Verification items for the finished model (mm, model axes). A direction names the side the tool comes from. Round coordinates to 2 decimals unless told otherwise and drop trailing zeros. Loops run counter-clockwise (first coordinate to the right, second up) from the corner with the lowest first, then second, coordinate; pieces in that order, holes last. Notation, with made-up numbers: M -32.5,31.25 L -25.5,31.25 A20 cw -25.5,64.25 Z; hole C 44,-14.5 d11. An arc over 180 degrees is marked long. One line per item, written item: value.
from build123d import *
from build123d.topology import SkipClean

# Parameters (mm, degrees)
SKETCH1_R           = 65
SKETCH1_R_2         = 5
SKETCH1_R_3         = 3
SKETCH1_R_4         = 1.55
BOSS_EXTRUDE1_DEPTH = 5
SKETCH2_R           = 14
CUT_EXTRUDE2_DEPTH  = 10
SKETCH3_R           = 2.25
SKETCH3_W           = 17.301764966
SKETCH3_H           = 25.534036418
CUT_EXTRUDE3_DEPTH  = 10
BOSS_EXTRUDE2_START = -27.5
SKETCH4_R           = 3
BOSS_EXTRUDE2_DEPTH = 22.5
SKETCH6_W           = 6
SKETCH6_H           = 20
CUT_EXTRUDE4_DEPTH  = 22.5
CUT_EXTRUDE5_REACH  = 101.575


with BuildPart() as part:
    # Sketch1 → Boss-Extrude1 (new body)
    with BuildSketch(Plane(origin=(0, 0, 0), x_dir=(1, 0, 0), z_dir=(0, 1, 0))):
        with Locations(Location((0, 0, 0), (0, 0, 270))):
            Circle(SKETCH1_R)
        with Locations(Location((0, 0, 0), (0, 0, 270))):
            Circle(SKETCH1_R_2, mode=Mode.SUBTRACT)
        with Locations(Location((0, 42.5, 0), (0, 0, 270))):
            Circle(SKETCH1_R_3, mode=Mode.SUBTRACT)
        with Locations(Location((42.5, 0, 0), (0, 0, 270))):
            Circle(SKETCH1_R_3, mode=Mode.SUBTRACT)
        with Locations(Location((0, -42.5, 0), (0, 0, 270))):
            Circle(SKETCH1_R_3, mode=Mode.SUBTRACT)
        with Locations(Location((-42.5, 0, 0), (0, 0, 270))):
            Circle(SKETCH1_R_3, mode=Mode.SUBTRACT)
        with Locations(Location((-42.5, -12.5, 0), (0, 0, 270))):
            Circle(SKETCH1_R_4, mode=Mode.SUBTRACT)
        with Locations(Location((-42.5, 12.5, 0), (0, 0, 270))):
            Circle(SKETCH1_R_4, mode=Mode.SUBTRACT)
        with Locations(Location((42.5, -12.5, 0), (0, 0, 90))):
            Circle(SKETCH1_R_4, mode=Mode.SUBTRACT)
        with Locations(Location((42.5, 12.5, 0), (0, 0, 90))):
            Circle(SKETCH1_R_4, mode=Mode.SUBTRACT)
    extrude(amount=BOSS_EXTRUDE1_DEPTH)

    # Sketch2 → Cut-Extrude2 (cut)
    with BuildSketch(Plane(origin=(0, 0, 0), x_dir=(-1, 0, 0), z_dir=(0, -1, 0))):
        with Locations(Location((-7.999467705, -0.092284522, 0), (0, 0, 90))):
            Circle(SKETCH2_R)
    extrude(amount=-CUT_EXTRUDE2_DEPTH, mode=Mode.SUBTRACT)

    # Sketch3 → Cut-Extrude3 (cut)
    with BuildSketch(Plane(origin=(0, 0, 0), x_dir=(-1, 0, 0), z_dir=(0, -1, 0))):
        with Locations(Location((-7.999467705, -17.592284522, 0), (0, 0, 90))):
            Circle(SKETCH3_R)
        with Locations(Location((-7.999467705, 17.407715478, 0), (0, 0, 90))):
            Circle(SKETCH3_R)
        with Locations((-18.812677283, 0)):
            Rectangle(SKETCH3_W, SKETCH3_H)
    extrude(amount=-CUT_EXTRUDE3_DEPTH, mode=Mode.SUBTRACT)

    # Sketch4 → Boss-Extrude2 (add)
    with BuildSketch(Plane(origin=(0, 5, 0), x_dir=(1, 0, 0), z_dir=(0, 1, 0)).offset(BOSS_EXTRUDE2_START)):
        Polygon((-7, 42.5), (-7, 22.5), (7, 22.5), (7, 42.5), (7, 48.5), (-7, 48.5), align=None)
        with Locations(Location((0, 42.5, 0), (0, 0, 270))):
            Circle(SKETCH4_R, mode=Mode.SUBTRACT)
    boss_extrude2 = extrude(amount=BOSS_EXTRUDE2_DEPTH)

    # Sketch6 → Cut-Extrude4 (cut)
    with BuildSketch(Plane(origin=(0, -22.5, 0), x_dir=(-1, 0, 0), z_dir=(0, -1, 0))):
        with Locations((0, 32.5)):
            Rectangle(SKETCH6_W, SKETCH6_H)
    cut_extrude4 = extrude(amount=-CUT_EXTRUDE4_DEPTH, mode=Mode.SUBTRACT)

    # Cut-Extrude5: up to this face of the body (flat: up to its plane)
    cut_extrude5_end = Plane(part.part.faces().sort_by_distance((-7, -11.25, -35.5))[0])
    # Sketch7 → Cut-Extrude5 (cut, up to the picked face)
    with BuildSketch(Plane(origin=(7, 0, 0), x_dir=(0, 0, -1), z_dir=(1, 0, 0)), mode=Mode.PRIVATE) as cut_extrude5_sk1:
        with BuildLine():
            Line((12.396013553, 0), (22.5, 0))
            ThreePointArc((22.5, 0), (30.667840434, -16.124515497), (48.5, -19.078784028))
            Line((48.5, -19.078784028), (48.5, -29.5))
            ThreePointArc((48.5, -29.5), (23.452348159, -23.31173437), (12.396013553, 0))
        make_face()
    cut_extrude5_tool1 = split(extrude(cut_extrude5_sk1.sketch, amount=-CUT_EXTRUDE5_REACH, mode=Mode.PRIVATE), bisect_by=cut_extrude5_end, keep=Keep.BOTH, mode=Mode.PRIVATE)
    # Sketch7 → Cut-Extrude5 (cut, up to the picked face)
    with BuildSketch(Plane(origin=(7, 0, 0), x_dir=(0, 0, -1), z_dir=(1, 0, 0)), mode=Mode.PRIVATE) as cut_extrude5_sk2:
        with BuildLine():
            ThreePointArc((42.5, -18.1), (45.6, -15), (42.5, -11.9))
            ThreePointArc((42.5, -11.9), (38.253817132, -11.116651072), (34.566666667, -8.869736311))
            ThreePointArc((34.566666667, -8.869736311), (30.189396423, -9.113673221), (30.433333333, -13.490943464))
            ThreePointArc((30.433333333, -13.490943464), (36.041520175, -16.908519697), (42.5, -18.1))
        make_face()
    cut_extrude5_tool2 = split(extrude(cut_extrude5_sk2.sketch, amount=-CUT_EXTRUDE5_REACH, mode=Mode.PRIVATE), bisect_by=cut_extrude5_end, keep=Keep.BOTH, mode=Mode.PRIVATE)
    cut_extrude5_1 = cut_extrude5_tool1.solids().sort_by(Axis((7, -17.317055, -28.895304), (-1, 0, 0)))[0]
    add(cut_extrude5_1, mode=Mode.SUBTRACT)
    cut_extrude5_2 = cut_extrude5_tool2.solids().sort_by(Axis((7, -13.514827, -37.337795), (-1, 0, 0)))[0]
    add(cut_extrude5_2, mode=Mode.SUBTRACT)
    cut_extrude5 = cut_extrude5_1 + cut_extrude5_2  # Cut-Extrude5 as one shape, for the pattern or mirror that repeats it

    # Mirror1: Boss-Extrude2, Cut-Extrude4, Cut-Extrude5 across plane
    with SkipClean():  # the faces are left unmerged after this step: merging them gives an invalid solid
        add(boss_extrude2.mirror(Plane.XY))
        add(cut_extrude4.mirror(Plane.XY), mode=Mode.SUBTRACT)
        add(cut_extrude5.mirror(Plane.XY), mode=Mode.SUBTRACT)


solid = part.part
(1) Sectioned sample at D-D on x = -42.5. Enter the section's corners in (y, z), and give its area (3 significant figures).
Completed:
outline: M 0,-49.18 L 5,-49.18 L 5,-14.05 L 0,-14.05 Z; M 0,-10.95 L 5,-10.95 L 5,-3 L 0,-3 Z; M 0,3 L 5,3 L 5,10.95 L 0,10.95 Z; M 0,14.05 L 5,14.05 L 5,49.18 L 0,49.18 Z
area: 431 mm^2
(2) Sectioned sample at B-B on x = 0. Enter the section's corners in (y, z).
Completed:
outline: M -19.77,-45.5 A20 ccw -19.08,-48.5 L 0,-48.5 L 0,-65 L 5,-65 L 5,-45.5 L -14.22,-45.5 A3.1 cw -15.78,-45.5 Z; M -19.77,45.5 L -15.78,45.5 A3.1 cw -14.22,45.5 L 5,45.5 L 5,65 L 0,65 L 0,48.5 L -19.08,48.5 A20 ccw Z; M 0,-39.5 L 5,-39.5 L 5,-11.4 L 0,-11.4 Z; M 0,11.58 L 5,11.58 L 5,39.5 L 0,39.5 Z
(3) Sectioned sample at C-C on z = 26. Enter the section's corners in (x, y), and give its area (3 significant figures).
Completed:
outline: M -59.57,0 L -7,0 L -7,-11.3 L -3,-11.3 L -3,0 L 3,0 L 3,-11.3 L 7,-11.3 L 7,0 L 59.57,0 L 59.57,5 L -59.57,5 Z
area: 686 mm^2
(4) Tool access check on faces 3 (the face through (21, 2, -12.767)), 4 (the face through (5.03, -11.14, 38.31)), 5 (the face through (-3, -7.9, 32.4)), 6 (the face through (3.2, -16, 30.5)). Record the directions out of +Z, -Z, +X, -X, +Y, -Y that give a thin tool (end or side, any length) a straight path to the whole face; none if there is none.
Completed:
face 3: +Y, -Y
face 4: +X, -X
face 5: -Y
face 6: +X, -X, -Y
(5) Depth check by flat-ended pin: pin 1 Ø4 at (x, z) = (42.5, 12.5) entering from -Y; pin 2 Ø6 at (y, z) = (-10, 37) entering from +X; pin 3 Ø5 at (y, z) = (-0.5, 41) entering from +X; pin 4 Ø3 at (x, z) = (-42.5, -12.5) entering from +Y. Enter the tip coordinate at first touch or a pass-through.
Completed:
pin 1: stops at y = 0
pin 2: stops at x = 7
pin 3: stops at x = 52.33
pin 4: passes through
(6) Thickness scan on L1, parallel to X at y = 3.5, z = 0; L2, parallel to X at y = -6.5, z = -30.5; L3, parallel to Z at x = -4, y = -14. Record the ranges inside material, lowest first. Write a range as from..to.
Completed:
L1: x = -65..-45.5, -39.5..-6, 27.46..39.5, 45.5..65
L2: x = -7..-3, 3..7
L3: z = -48.5..-45.43, -31.03..-28.22, 28.22..31.03, 45.43..48.5
(7) Sectioned sample at A-A on y = -1.5. Enter the section's corners in (x, z).
Completed:
outline: M -7,-48.5 L 7,-48.5 L 7,-22.56 L 3,-22.56 L 3,-42.5 A3 cw -3,-42.5 L -3,-22.56 L -7,-22.56 Z; M -7,22.56 L -3,22.56 L -3,42.5 A3 cw 3,42.5 L 3,22.56 L 7,22.56 L 7,48.5 L -7,48.5 Z
(8) Mould release check, pull along Z, two halves, no side actions. Record for faces 1 (the face through (0.1, -18.4, -45.5)), 2 (the face through (-7, -8, 39)): +Z half, -Z half, draft (parallel to the pull), parting line (faces both ways), or undercut.
Completed:
face 1: undercut
face 2: draft
